Verification items for the finished model (mm, model axes). Face numbers are marked on the shaded views. A direction names the side the tool comes from. Coordinates: 2 decimals unless noted, no trailing zeros. Order: outer loops, then holes, each group sorted by start corner. A loop starts at its lowest first (then second) coordinate and runs counter-clockwise, first axis right, second up.
Q1. Cross-section at D-D, the plane z = 3.5. Record the boundary of the cut face in (x, y), and give its area (3 significant figures).
Q2. Depth check by flat-ended pin: P1, Ø5, axis at x = -6.5, z = 3, coming from the +Y side; P2, Ø2, axis at x = 4, z = 2.5, coming from the -Y side; P3, Ø4, axis at y = 6.5, z = 9.5, coming from the +X side; P4, Ø11, axis at x = 0, y = 0, coming from the +Z side. Enter the tip coordinate at first touch or a pass-through.
Q3. Cross-section at A-A, the plane x = 0. Record the boundary of the cut face in (y, z), and give its area (3 significant figures).
Q4. Draft check along X on the marked faces 3, 4 and 5. Enter one of: pulls with the +X half, pulls with the -X half, needs draft (parallel to the pull), parting line crosses it, or undercut.
Q5. Cross-section at C-C, the plane z = 8. Record the boundary of the cut face in (x, y), and give its area (3 significant figures).
Q6. Thickness scan on line 1 (Y direction, x = 0, z = 9.25); line 2 (Y direction, x = 0, z = 4); line 3 (X direction, y = 6.25, z = 6). Record the ranges inside material, lowest first.
Q7. Set-up check for the marked faces 1 and 2: record each of +Z, -Z, +X, -X, +Y, -Y from which the full face is reachable in a straight line by a thin tool's end or side.
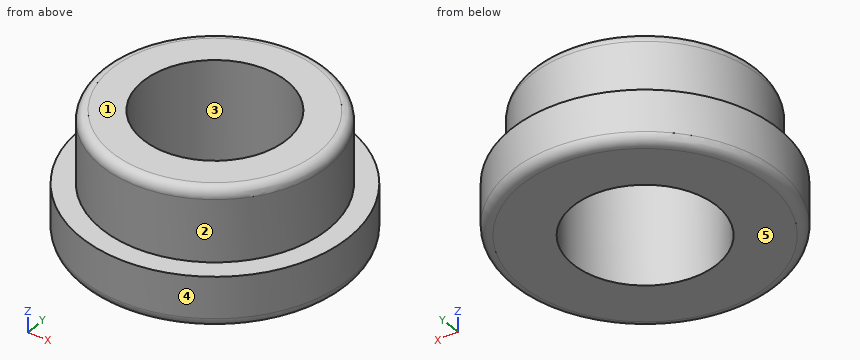
from build123d import *

# Parameters (mm, degrees)
F0_R           = 13
F1_DEPTH       = 5
F2_R           = 11
F3_DEPTH       = 7
F5_D           = 14
F5_CBORE_D     = 14
F5_CBORE_DEPTH = 14
F6_R           = 0.965685
F7_R           = 0.965685


with BuildPart() as f1:
    # F0 (on Top) → F1 (new body)
    with BuildSketch(Plane.XY):
        Circle(F0_R)
    extrude(amount=F1_DEPTH)

    # F2 (on face) → F3 (join)
    with BuildSketch(Plane.XY.offset(5)):
        Circle(F2_R)
    extrude(amount=F3_DEPTH)

    # F5 (through all)
    with Locations(Plane.XY.offset(12)):
        with Locations((0, 0)):
            CounterBoreHole(F5_D / 2, F5_CBORE_D / 2, F5_CBORE_DEPTH)

    # F6
    f6_edges = [f1.edges().sort_by_distance(p)[0] for p in [
        (-11, 0, 12),
    ]]
    fillet(f6_edges, radius=F6_R)

    # F7
    f7_edges = [f1.edges().sort_by_distance(p)[0] for p in [
        (-13, 0, 0),
    ]]
    fillet(f7_edges, radius=F7_R)


solid = f1.part
Check values:
1. outline: circle Ø26 at (0, 0); hole circle Ø14 at (0, 0)
1. area: 377 mm2
2. P1: stops at y = 12.37
2. P2: stops at y = -12.65
2. P3: stops at x = 10.04
2. P4: passes through
3. outline: (-13, 0.97) arc R0.97 ccw to (-12.03, 0) - (-7, 0) - (-7, 12) - (-10.03, 12) arc R0.97 ccw to (-11, 11.03) - (-11, 5) - (-13, 5) - close; (7, 0) - (12.03, 0) arc R0.97 ccw to (13, 0.97) - (13, 5) - (11, 5) - (11, 11.03) arc R0.97 ccw to (10.03, 12) - (7, 12) - close
3. area: 115 mm2
4. face 3: undercut
4. face 4: parting line crosses it
4. face 5: needs draft
5. outline: circle Ø22 at (0, 0); hole circle Ø14 at (0, 0)
5. area: 226 mm2
6. line 1: y = -11 to -7, 7 to 11
6. line 2: y = -13 to -7, 7 to 13
6. line 3: x = -9.05 to -3.15, 3.15 to 9.05
7. face 1: +Z, +X, -X, +Y, -Y
7. face 2: +Z
